The listing builds one solid part. Answer for the finished solid, in the listing's coordinates (mm). Face numbers are marked on the shaded views. A direction names the side the tool comes from. Round coordinates to 2 decimals unless told otherwise and drop trailing zeros. Order: outer loops, then holes, each group sorted by start corner. A loop starts at its lowest first (then second) coordinate and runs counter-clockwise, first axis right, second up. Notation, with made-up numbers: (31, 77.25) - (46, 77.25) arc R23 cw to (46, 100.25) - close; hole circle Ø11 at (6, -16.75). An arc over 180 degrees is marked (long way). One line per item, written item: value. Start each with the question number.
1. Section A-A, the plane z = 32 is taken. Give the vertices of the cut face in (x, y), then the cut area to 3 significant figures.
2. Section C-C, the plane x = -9 is taken. Give the vertices of the cut face in (y, z).
3. Flat-ended cylindrical pins translate along their axes: P1, Ø1.5, axis at y = -498.5, z = 24, coming from the -X side; P2, Ø2.5, axis at y = -500, z = 32, coming from the +X side; P3, Ø6.5, axis at y = -496.5, z = 18, coming from the -X side. Find the tip coordinate at first contact, or state that the pin passes through.
4. Section D-D, the plane y = -496 is taken. Give the vertices of the cut face in (x, z).
5. For a pull along Z with two mould halves and no side action, classify the marked faces 3, 4, 5 and 6 as released by +Z, released by -Z, zero draft, split by the parting line, or undercut.
6. A tool of negligible diameter and unlimited length cuts with its end or side. For the marked faces 1 and 2, from which of +Z, -Z, +X, -X, +Y, -Y can it reach the whole face along a straight path? Write none if from no direction.
7. Section B-B, the plane x = -13 is taken. Give the vertices of the cut face in (y, z) (3 decimals).
8. Straight lines are drawn through the part: line 1 (X direction, y = -496, z = 36.5); line 2 (Y direction, x = 12, z = 34.25); line 3 (Y direction, x = 13.75, z = 32). For each, find the intervals that lie inside material, in ascending order.
from build123d import *

# Parameters (mm, degrees)
PAD026_DEPTH            = 8
SKETCH051_R             = 2
POCKET019_DEPTH         = 8
SKETCH052_R             = 2
POCKET020_DEPTH         = 8
BODY020_PLACEMENT_ANGLE = 180


with BuildPart() as part:
    # Sketch050 → Pad026 (new body, symmetric)
    with BuildSketch(Plane.XZ):
        Polygon((-16, 38), (16, 38), (16, 26), (12, 20.5), (12, 14.5), (16, 9), (16, 4), (-16, 4), (-16, 9), (-12, 14.5), (-12, 20.5), (-16, 26), align=None)
    extrude(amount=PAD026_DEPTH, both=True)

    # Sketch051 (on Face1 of Pad026) → Pocket019 (cut)
    with BuildSketch(Plane(origin=(0, 0, 38), x_dir=(-1, 0, 0), z_dir=(0, 0, 1))):
        with Locations((-12, 4)):
            Circle(SKETCH051_R)
        with Locations((-12, -4)):
            Circle(SKETCH051_R)
        with Locations((12, -4)):
            Circle(SKETCH051_R)
        with Locations((12, 4)):
            Circle(SKETCH051_R)
    extrude(amount=-POCKET019_DEPTH, mode=Mode.SUBTRACT)

    # Sketch052 (on Face2 of Pocket019) → Pocket020 (cut)
    with BuildSketch(Plane(origin=(-16, 0, 0), x_dir=(0, 0, -1), z_dir=(-1, 0, 0))):
        with Locations((-32, 0)):
            Circle(SKETCH052_R)
    pocket020 = extrude(amount=-POCKET020_DEPTH, mode=Mode.SUBTRACT)

    # Mirrored001: Pocket020 across YZ
    add(pocket020.mirror(Plane.YZ), mode=Mode.SUBTRACT)


with BuildPart() as part_1:
    # Body020 placement: moved
    add(part.part.moved(Location((0, -500, 0))).rotate(Axis((0, -500, 0), (0, 0, 1)), BODY020_PLACEMENT_ANGLE))


solid = part_1.part
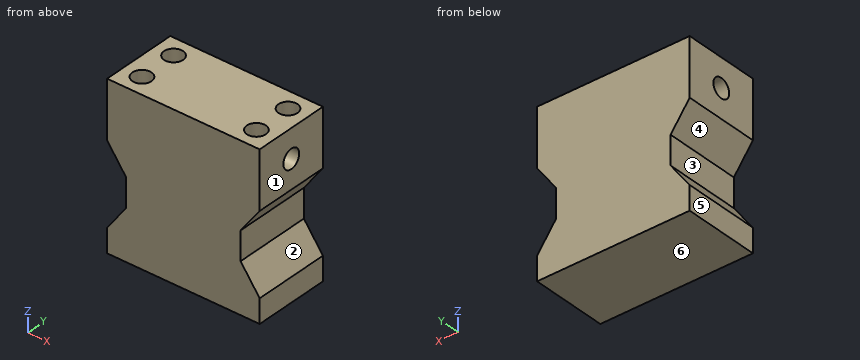
Answer list:
1. outline: (-16, -508) - (16, -508) - (16, -502) - (8, -502) - (8, -498) - (16, -498) - (16, -492) - (-16, -492) - (-16, -498) - (-8, -498) - (-8, -502) - (-16, -502) - close; hole circle Ø4 at (-12, -504); hole circle Ø4 at (-12, -496); hole circle Ø4 at (12, -504); hole circle Ø4 at (12, -496)
1. area: 398 mm²
2. outline: (-508, 4) - (-492, 4) - (-492, 38) - (-508, 38) - close; hole circle Ø4 at (-500, 32)
3. P1: stops at x = -15.09
3. P2: stops at x = 8
3. P3: stops at x = -12.55
4. outline: (-16, 4) - (16, 4) - (16, 9) - (12, 14.5) - (12, 20.5) - (16, 26) - (16, 38) - (14, 38) - (14, 30) - (10, 30) - (10, 38) - (-10, 38) - (-10, 30) - (-14, 30) - (-14, 38) - (-16, 38) - (-16, 26) - (-12, 20.5) - (-12, 14.5) - (-16, 9) - close
5. face 3: undercut
5. face 4: undercut
5. face 5: zero draft
5. face 6: released by -Z
6. face 1: +Z, -Z, +X, +Y, -Y
6. face 2: +X, +Y, -Y
7. outline: (-508, 4) - (-492, 4) - (-492, 13.125) - (-508, 13.125) - close; (-508, 21.875) - (-492, 21.875) - (-492, 38) - (-494.268, 38) - (-494.268, 30) - (-497.732, 30) - (-497.732, 38) - (-502.268, 38) - (-502.268, 30) - (-505.732, 30) - (-505.732, 38) - (-508, 38) - close; hole circle Ø4 at (-500, 32)
8. line 1: x = -16 to -14, -10 to 10, 14 to 16
8. line 2: y = -508 to -506, -502 to -498, -494 to -492
8. line 3: y = -508 to -504.97, -503.03 to -502, -498 to -496.97, -495.03 to -492
